Solid Edge part; units mm, degrees
sketch "Sketch1" plane through (0, 0, 0) normal (0, -1, 0) x (1, 0, 0)
  line L0 (17.4625, 7.2332) -> (7.2332, 17.4625)
  line L1 (7.2332, 17.4625) -> (-7.2332, 17.4625)
  line L2 (-7.2332, 17.4625) -> (-17.4625, 7.2332)
  line L3 (-17.4625, 7.2332) -> (-17.4625, -7.2332)
  line L4 (-17.4625, -7.2332) -> (-7.2332, -17.4625)
  line L5 (-7.2332, -17.4625) -> (7.2332, -17.4625)
  line L6 (7.2332, -17.4625) -> (17.4625, -7.2332)
  line L7 (17.4625, -7.2332) -> (17.4625, 7.2332)
extrude "Protrusion1" add sketch "Sketch1" against normal blind 6.35
sketch "Sketch2" plane through (0, 6.35, 0) normal (0, 1, 0) x (-1, 0, 0)
  circle A0 centre (0, 0) radius 12.7
extrude "ExtrudedProtrusion_2" add sketch "Sketch2" along normal blind 15.875
sketch "Sketch3" plane through (0, 0, 0) normal (-1, 0, 0) x (0, -1, 0)
  line L0 (44.45, 19.05) -> (44.45, 22.225)
  line L1 (0, 15.875) -> (44.45, 22.225)
  line L2 (0, 0) -> (0, 15.875)
  line L3 (6.35, 0) -> (0, 0)
  line L4 (6.35, 0) -> (6.35, 13.6071)
  line L5 (6.35, 13.6071) -> (44.45, 19.05)
revolve "RevolvedProtrusion1" add sketch "Sketch3" angle 360 about axis through (0, -44.45, 0) along (0, 1, 0)
fillet "Round_1" radius 1.5875 2 edges at (0, -44.45, -22.225) (0, -44.45, -19.05)
cosmetic_thread "Thread1"
sketch "Sketch4" plane through (0, 22.225, 0) normal (0, 1, 0) x (-1, 0, 0)
  line L0 (-9.525, -3.175) -> (9.525, -3.175)
  line L1 (9.525, -3.175) -> (9.525, 3.175)
  line L2 (9.525, 3.175) -> (-9.525, 3.175)
  line L3 (-9.525, 3.175) -> (-9.525, -3.175)
  dimension "D1" = 9.525
  dimension "D2" = 9.525
extrude "ExtrudedProtrusion_3" add sketch "Sketch4" along normal blind 6.35
sketch "Sketch5" plane through (0, 25.4, -3.175) normal (0, 0, -1) x (0, -1, 0)
  line L0 (-3.175, 9.525) -> (0, 9.525)
  line L1 (0, 9.525) -> (0, -9.525)
  line L2 (0, -9.525) -> (-3.175, -9.525)
  line L3 (-3.175, -9.525) -> (-3.175, 9.525)
extrude "ExtrudedProtrusion_4" add sketch "Sketch5" along normal blind 6.35
properties material "ABS Plastic, high impact"
Design review of the part built by this model. Coordinates are the model's own, in mm. A direction names the side the tool comes from. Coordinates: 2 decimals unless noted, no trailing zeros. Loops run counter-clockwise (first coordinate to the right, second up) from the corner with the lowest first, then second, coordinate; pieces in that order, holes last.
Q1. To check wall thickness, follow line 1 (X direction, y = 12.5, z = 11); line 2 (Z direction, x = 12, y = -25.5); line 3 (X direction, y = -7, z = 10). State the ranges of each line that lie inside material, in increasing order.
Reported:
line 1: x = -6.35 to 6.35
line 2: z = -15.39 to -11.09, 11.09 to 15.39
line 3: x = -13.59 to -9.36, 9.36 to 13.59
Q2. We need section A-A on y = 2. State the section outline as (x, z) points.
Reported:
outline: (-17.46, -7.23) - (-7.23, -17.46) - (7.23, -17.46) - (17.46, -7.23) - (17.46, 7.23) - (7.23, 17.46) - (-7.23, 17.46) - (-17.46, 7.23) - close
Q3. Tool access review of faces 1 (the face through (12.419, 3.131, 12.276)), 2 (the face through (-14, 0, -8)), 3 (the face through (0, 3, -17.462)), 4 (the face through (9.525, 26, -2)), 5 (the face through (-12.276, 3.131, 12.419)): name each direction out of +Z, -Z, +X, -X, +Y, -Y from which nothing blocks a thin tool from reaching the whole face with its end or side.
Reported:
face 1: +Z, +X, +Y
face 2: none
face 3: -Z, +X, -X, +Y
face 4: +Z, -Z, +X, +Y
face 5: +Z, -X, +Y
Q4. The part is to be moulded in two halves that separate along Z. For faces 6 (the face through (0, 24, -3.175)), 7 (the face through (0, -6.35, 0)), 8 (the face through (15.31, -20.89, -3.4)), 9 (the face through (0, 22.225, 5)), say which applies: +Z half, -Z half, draft (parallel to the pull), parting line (faces both ways), or undercut.
Reported:
face 6: -Z half
face 7: undercut
face 8: undercut
face 9: draft
Q5. We need section D-D on y = -10.5. State the section outline as (x, z) points (3 decimals).
Reported:
outline: circle Ø34.75 at (0, 0); hole circle Ø28.4 at (0, 0)
Q6. For pin 1 (4 mm diameter, centred on y = -34.5, z = -17.5, fed in from -X); pin 2 (5 mm diameter, centred on y = 24, z = -1.5, fed in from -X); pin 3 (5 mm diameter, centred on y = 8.5, z = 4.5, fed in from -X); pin 4 (12 mm diameter, centred on x = -14, z = -12.5, fed in from -Y), all flat-tipped, find the tip position at first contact; note any pin that passes through.
Reported:
pin 1: stops at x = -13.92
pin 2: stops at x = -12.7
pin 3: stops at x = -17.46
pin 4: stops at y = -44.45
